Job drawing, mm, ordinate dimensions from the low corner. One solid piece. A direction names the side the tool comes from. Round coordinates to 2 decimals unless told otherwise and drop trailing zeros. Order: outer loops, then holes, each group sorted by start corner. A loop starts at its lowest first (then second) coordinate and runs counter-clockwise, first axis right, second up. Notation, with made-up numbers: (81, 16.5) -> (85, 16.5) arc R16 ccw to (85, 32.5) -> close; hole circle Ø11 at (13.5, 75). An arc over 180 degrees is marked (long way). Return JSON: item names as keys, results as strings. Group by question number.
Q1. Flat gauge pins, fed straight in: pin 1 (4 mm diameter, centred on x = 44, y = 7.5, fed in from +Z); pin 2 (1.5 mm diameter, centred on x = 35.5, z = 13, fed in from -Y); pin 3 (12 mm diameter, centred on y = 15, z = 18, fed in from -X). Where does each tip first touch, or does it go through?
Q2. Cut at D-D (z = 23). Write the cut outline in (x, y).
Q3. Probe line 1 along Z through (x, y) = (7.5, 12); line 2 along X through (y, z) = (15, 16.5); line 3 along Y through (x, z) = (66.5, 4). List the from-to ranges inside material, lowest first.
Q4. Cut at A-A (y = 22.5). Write the cut outline in (x, z), then the cut area to 3 significant figures.
Q5. Which spindle directions (+Z, -Z, +X, -X, +Y, -Y) get a long thin tool onto all of the face, cutting with end or side? Do the marked faces 4, 5, 6 and 7. Say none if no direction does.
Q6. Cut at C-C (y = 5). Write the cut outline in (x, z), then the cut area to 3 significant figures.
Q7. Mould opens along X. For the marked faces 1, 2 and 3 say: +X half, -X half, draft (parallel to the pull), parting line (faces both ways), or undercut.
Q8. Cut at B-B (z = 4.5). Write the cut outline in (x, y).
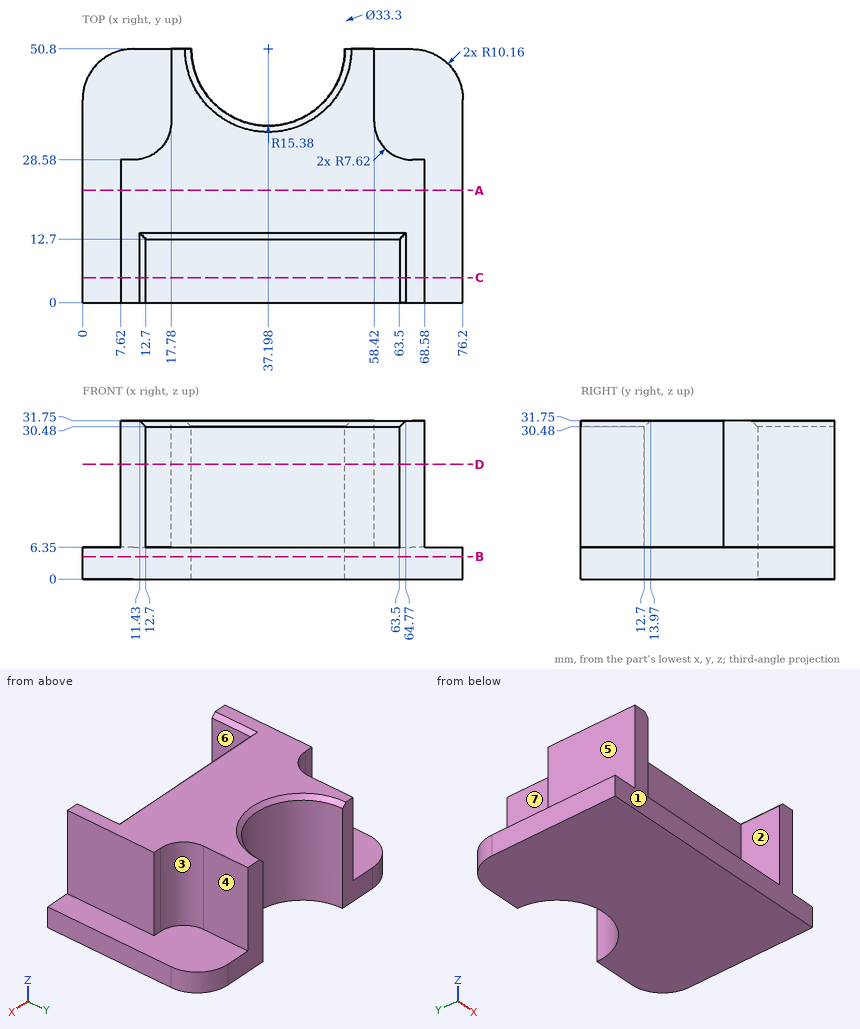
Solution:
{
 "1": {"pin 1": "stops at z = 6.35", "pin 2": "stops at y = 12.7", "pin 3": "stops at x = 7.62"},
 "2": {"outline": "(7.62, 0) -> (12.7, 0) -> (12.7, 12.7) -> (63.5, 12.7) -> (63.5, 0) -> (68.58, 0) -> (68.58, 28.58) -> (66.04, 28.58) arc R7.62 cw to (58.42, 36.2) -> (58.42, 50.8) -> (52.58, 50.8) arc R15.38 cw to (21.82, 50.8) -> (17.78, 50.8) -> (17.78, 36.2) arc R7.62 cw to (10.16, 28.58) -> (7.62, 28.58) -> close"},
 "3": {"line 1": "z = 0 to 6.35", "line 2": "x = 7.62 to 68.58", "line 3": "y = 0 to 50.79"},
 "4": {"outline": "(0, 0) -> (76.2, 0) -> (76.2, 6.35) -> (68.58, 6.35) -> (68.58, 31.75) -> (7.62, 31.75) -> (7.62, 6.35) -> (0, 6.35) -> close", "area": "2,030 mm²"},
 "5": {"face 4": "+Z, +X, +Y", "face 5": "+Z, -X, +Y, -Y", "face 6": "+Z, -Y", "face 7": "+Z, -X, +Y"},
 "6": {"outline": "(0, 0) -> (76.2, 0) -> (76.2, 6.35) -> (68.58, 6.35) -> (68.58, 31.75) -> (64.77, 31.75) -> (63.5, 30.48) -> (63.5, 6.35) -> (12.7, 6.35) -> (12.7, 30.48) -> (11.43, 31.75) -> (7.62, 31.75) -> (7.62, 6.35) -> (0, 6.35) -> close", "area": "740 mm²"},
 "7": {"face 1": "draft", "face 2": "undercut", "face 3": "+X half"},
 "8": {"outline": "(0, 0) -> (76.2, 0) -> (76.2, 40.64) arc R10.16 ccw to (66.04, 50.8) -> (52.58, 50.8) arc R15.38 cw to (21.82, 50.8) -> (10.16, 50.8) arc R10.16 ccw to (0, 40.64) -> close"}
}
